from build123d import *

# Parameters (mm, degrees)
CROQUIS2_R = 3.75


with BuildPart() as part:
    # Barrer1: sweep along a path in Croquis1
    with BuildLine(Plane(origin=(0, 0, 0), x_dir=(1, 0, 0), z_dir=(0, 1, 0))) as barrer1_path:
        Line((0, 0), (0, 20))
        ThreePointArc((0, 20), (2.928932188, 27.071067812), (10, 30))
        Line((10, 30), (136.4548, 30))
        ThreePointArc((136.4548, 30), (143.525867812, 27.071067812), (146.4548, 20))
        Line((146.4548, 20), (146.4548, 0))
    # Croquis2 → Barrer1 (sweep)
    with BuildSketch(Plane.XY):
        Circle(CROQUIS2_R)
    sweep(path=barrer1_path.line)


solid = part.part
Verification items for the finished model (mm, model axes). A direction names the side the tool comes from. Give positions to 0.01 mm unless a question says otherwise; leave off trailing zeros. Write each loop counter-clockwise with the first axis right and the second up, starting at its lowest first coordinate (ties: lowest second). Pieces come first, ordered by that corner, then holes. Notation, with made-up numbers: M 60,-11.75 L 70,-11.75 A10 ccw 70,-0.75 Z; hole C 55,31.25 d1. An arc over 180 degrees is marked long. Use CSV: the item, a comma, the result in double quotes.
1) Cross-section at B-B (z = -3.5). Enter the section's corners in (x, y), plus the area to 3 significant figures.
Final values:
outline,"C 0,0 d7.5; C 146.45,0 d7.5"
area,"88.4 mm²"
2) Cross-section at A-A (y = 0). Enter the section's corners in (x, z), plus the area to 3 significant figures.
Final values:
outline,"M -3.75,-20 A13.75 ccw 10,-33.75 L 136.45,-33.75 A13.75 ccw 150.2,-20 L 150.2,0 L 142.7,0 L 142.7,-20 A6.25 cw 136.45,-26.25 L 10,-26.25 A6.25 cw 3.75,-20 L 3.75,0 L -3.75,0 Z"
area,"1,480 mm²"
3) Cross-section at C-C (x = 110.5). Enter the section's corners in (y, z).
Final values:
outline,"C 0,-30 d7.5"
4) Go/stop test with flat-tipped pins: pin 1 Ø1 at (x, y) = (24, -3) entering from +Z; pin 2 Ø3 at (y, z) = (2.5, -27) entering from -X; pin 3 Ø1.5 at (x, y) = (45, -1.5) entering from -Z. Record where each tip stops, or that it passes through.
Final values:
pin 1,"z = -27.2"
pin 2,"x = -2.08"
pin 3,"z = -33.67"
5) Material ranges on line 1 along X through (y, z) = (-0.25, -10); line 2 along Z through (x, y) = (22, -0.25); line 3 along X through (y, z) = (3.25, -13), recorded low to high.
Final values:
line 1,"-3.74 to 3.74, 142.71 to 150.2"
line 2,"-33.74 to -26.26"
line 3,"-1.87 to 1.87, 144.58 to 148.33"
6) Access from +Z, -Z, +X, -X, +Y, -Y to the whole of each face (thin tool, end or side, straight path). Record for faces 1 (the face through (147, 0, 0)), 2 (the face through (74.113, -0.165, -33.746)), 3 (the face through (150.2, -0.2, -9.9)).
Final values:
face 1,"+Z, +X, -X, +Y, -Y"
face 2,"none"
face 3,"+Z"
7) Release check for a two-part mould opening along X. For faces 4 (the face through (0, 0, 0)), 5 (the face through (-3.746, -0.165, -10.14)) record: released by +X, released by -X, zero draft, split by the parting line, or undercut.
Final values:
face 4,"zero draft"
face 5,"undercut"
